```python
from build123d import *

# Parameters (mm, degrees)
SKETCH1_R               = 9.36
SKETCH1_R_2             = 7.99
EXTRUDE1_DEPTH          = 457.2
SKETCH2_R               = 9.525
CUT_EXTRUDE1_DEPTH      = 10.36
CUT_EXTRUDE1_DEPTH_BACK = 10.36
SKETCH3_R               = 9.525
CUT_EXTRUDE2_DEPTH      = 10.3600001
CUT_EXTRUDE2_DEPTH_BACK = 10.3600001
SKETCH5_R               = 1.55
CUT_EXTRUDE3_DEPTH      = 10.3600001
CUT_EXTRUDE3_DEPTH_BACK = 10.3600001


with BuildPart() as part:
    # Sketch1 → Extrude1 (new body)
    with BuildSketch(Plane.XY):
        Circle(SKETCH1_R)
        Circle(SKETCH1_R_2, mode=Mode.SUBTRACT)
    extrude(amount=EXTRUDE1_DEPTH)

    # Sketch2 → Cut-Extrude1 (cut, two sides)
    with BuildSketch(Plane(origin=(0, 0, 0), x_dir=(0, 0, -1), z_dir=(1, 0, 0))) as cut_extrude1_sk:
        Circle(SKETCH2_R)
    extrude(amount=CUT_EXTRUDE1_DEPTH, mode=Mode.SUBTRACT)
    extrude(cut_extrude1_sk.sketch, amount=-CUT_EXTRUDE1_DEPTH_BACK, mode=Mode.SUBTRACT)

    # Sketch3 → Cut-Extrude2 (cut, two sides)
    with BuildSketch(Plane(origin=(0, 0, 0), x_dir=(0, 0, -1), z_dir=(1, 0, 0))) as cut_extrude2_sk:
        with Locations((-457.2, 0)):
            Circle(SKETCH3_R)
    extrude(amount=CUT_EXTRUDE2_DEPTH, mode=Mode.SUBTRACT)
    extrude(cut_extrude2_sk.sketch, amount=-CUT_EXTRUDE2_DEPTH_BACK, mode=Mode.SUBTRACT)

    # Sketch5 → Cut-Extrude3 (cut, two sides)
    with BuildSketch(Plane(origin=(0, 0, 0), x_dir=(1, 0, 0), z_dir=(0, 1, 0))) as cut_extrude3_sk:
        with Locations((0, -441.33)):
            Circle(SKETCH5_R)
        with Locations((0, -15.88)):
            Circle(SKETCH5_R)
    extrude(amount=CUT_EXTRUDE3_DEPTH, mode=Mode.SUBTRACT)
    extrude(cut_extrude3_sk.sketch, amount=-CUT_EXTRUDE3_DEPTH_BACK, mode=Mode.SUBTRACT)


solid = part.part
```
Build history of the part. All positions in model axes, mm. Round coordinates to 2 decimals unless told otherwise and drop trailing zeros. Order: outer loops, then holes, each group sorted by start corner. A loop starts at its lowest first (then second) coordinate and runs counter-clockwise, first axis right, second up. Notation, with made-up numbers: (54.5, -3) -> (63.5, -3) arc R12 ccw to (63.5, 6) -> close; hole circle Ø9 at (8, 31). An arc over 180 degrees is marked (long way). Answer in a Markdown table with one row per item.
1) Wall check: L1, parallel to X at y = 1, z = 357.5; L2, parallel to Y at x = -0.5, z = 84; L3, parallel to Z at x = 0, y = 8.65. Give the ranges that are in metal, low to high.
Values:
| item | result |
|---|---|
| L1 | -9.31 to -7.93, 7.93 to 9.31 |
| L2 | -9.35 to -7.97, 7.97 to 9.35 |
| L3 | 3.99 to 14.33, 17.43 to 439.78, 442.88 to 453.21 |
2) Pin check, flat tips, straight feed: P1, Ø1, axis at x = -5.5, z = 117.5, coming from the +Y side; P2, Ø6, axis at x = -3.5, y = -5.5, coming from the -Z side; P3, Ø3, axis at x = 0.5, y = -7, coming from the +Z side. Stop position of each tip, or through.
Values:
| item | result |
|---|---|
| P1 | y = 7.91 |
| P2 | z = 4.3 |
| P3 | z = 452.9 |
3) Band-saw the part on A-A on y = -4.75. Give the cut face in (x, z), and give its area (3 significant figures).
Values:
| item | result |
|---|---|
| outline | (-8.07, 8.26) -> (-6.42, 8.26) -> (-6.42, 448.94) -> (-8.07, 448.94) -> close; (6.42, 8.26) -> (8.07, 8.26) -> (8.07, 448.94) -> (6.42, 448.94) -> close |
| area | 1,450 mm2 |
4) Band-saw the part on C-C on z = 203. Give the cut face in (x, y).
Values:
| item | result |
|---|---|
| outline | circle Ø18.72 at (0, 0); hole circle Ø15.98 at (0, 0) |
5) Band-saw the part on B-B on x = 4.75. Give the cut face in (y, z) (3 decimals), and give its area (3 significant figures).
Values:
| item | result |
|---|---|
| outline | (-8.065, 5.067) arc R9.525 cw to (-6.425, 7.032) -> (-6.425, 450.168) arc R9.525 cw to (-8.065, 452.133) -> close; (6.425, 7.032) arc R9.525 cw to (8.065, 5.067) -> (8.065, 452.133) arc R9.525 cw to (6.425, 450.168) -> close |
| area | 1,460 mm2 |
6) Mould opens along Y. For faces 1 (the cylindrical face through (-7.428, -5.695, 225.424)), 2 (the cylindrical face through (2.72, 7.63, 5.7)), 3 (the cylindrical face through (-0.738, 8.111, 452.207)) say: released by +Y, released by -Y, zero draft, split by the parting line, or undercut.
Values:
| item | result |
|---|---|
| face 1 | split by the parting line |
| face 2 | undercut |
| face 3 | undercut |
